Autodesk Inventor part; units mm, degrees
ref_plane "YZ Plane" through (0, 0, 0) normal (1, 0, 0) x (0, 1, 0)
ref_plane "XZ Plane" through (0, 0, 0) normal (0, 1, 0) x (-1, 0, 0)
ref_plane "XY Plane" through (0, 0, 0) normal (0, 0, 1) x (1, 0, 0)
sketch "Sketch13" plane through (0, 0, 0) normal (0, 0, 1) x (1, 0, 0)
  line L0 (-50, 45) -> (50, 45)
  line L1 (50, 45) -> (50, 0)
  line L2 (50, 0) -> (-50, 0)
  line L3 (-50, 0) -> (-50, 45)
  line L4 (-50, 45) -> (50, 0) construction
  line L5 (50, 45) -> (-50, 0) construction
  point P0 (0, 0)
  point P1 (0, 22.5)
  dimension "d42" = 100
  dimension "d43" = 45
extrude "Extrusion11" add sketch "Sketch13" along normal blind 50
sketch "Sketch14" plane through (0, 0, 50) normal (0, 0, 1) x (1, 0, 0)
  circle A0 centre (0, 0) radius 40
  dimension "d46" = 80
extrude "Extrusion12" cut sketch "Sketch14" against normal blind 50
sketch "Sketch15" plane through (0, 0, 50) normal (0, 0, 1) x (1, 0, 0)
  point P0 (0, 0)
properties part number "pipe_holder_v02"
For this review, take the finished solid that the model builds, in its own axes (mm). Coordinates: 2 decimals unless noted, no trailing zeros. Loops run counter-clockwise (first coordinate to the right, second up) from the corner with the lowest first, then second, coordinate; pieces in that order, holes last. Notation, with made-up numbers: (85, -26.75) -> (133, -26.75) arc R9 ccw to (133, -17.75) -> close; hole circle Ø9 at (-39.75, 12.5). An arc over 180 degrees is marked (long way). Write each question's results on one line, items separated by ' | '.
Q1. To check wall thickness, follow line 1 along X through (y, z) = (12, 13.5); line 2 along X through (y, z) = (19, 23); line 3 along Y through (x, z) = (24.5, 19). State the ranges of each line that lie inside material, in increasing order. Write a range as [from, to].
Taken from the geometry:
line 1: [-50, -38.16], [38.16, 50] | line 2: [-50, -35.2], [35.2, 50] | line 3: [31.62, 45]
Q2. Add section B-B, the plane z = 27.5. State the section outline as (x, y) points, then the cut area to 3 significant figures.
Taken from the geometry:
outline: (-50, 0) -> (-40, 0) arc R40 cw to (40, 0) -> (50, 0) -> (50, 45) -> (-50, 45) -> close | area: 1,990 mm²
Q3. Mouldability with a two-part tool opening along X and no side actions: class faces 1 (the flat face through (-1, 43, 0)), 2 (the cylindrical face through (0.88, 39.99, 25.35)), 3 (the flat face through (50, 23, 25)) as +X half, -X half, draft (parallel to the pull), parting line (faces both ways), or undercut.
Taken from the geometry:
face 1: draft | face 2: undercut | face 3: +X half
Q4. For pin 1 Ø1 at (x, y) = (37.5, 16) entering from -Z; pin 2 Ø1.5 at (x, z) = (-6.5, 42.5) entering from -Y; pin 3 Ø12 at (x, y) = (26.5, 10.5) entering from -Z; pin 4 Ø12 at (x, z) = (-0.5, 20) entering from -Y, all flat-tipped, find the tip position at first contact; note any pin that passes through.
Taken from the geometry:
pin 1: z = 0 | pin 2: y = 39.34 | pin 3: through | pin 4: y = 39.47
Q5. Add section C-C, the plane x = 0. State the section outline as (y, z) points, then the cut area to 3 significant figures.
Taken from the geometry:
outline: (40, 0) -> (45, 0) -> (45, 50) -> (40, 50) -> close | area: 250 mm²
Q6. Add section D-D, the plane y = 5. State the section outline as (x, z) points.
Taken from the geometry:
outline: (-50, 0) -> (-39.69, 0) -> (-39.69, 50) -> (-50, 50) -> close; (39.69, 0) -> (50, 0) -> (50, 50) -> (39.69, 50) -> close
Q7. Add section A-A, the plane y = 32. State the section outline as (x, z) points, then the cut area to 3 significant figures.
Taken from the geometry:
outline: (-50, 0) -> (-24, 0) -> (-24, 50) -> (-50, 50) -> close; (24, 0) -> (50, 0) -> (50, 50) -> (24, 50) -> close | area: 2,600 mm²
